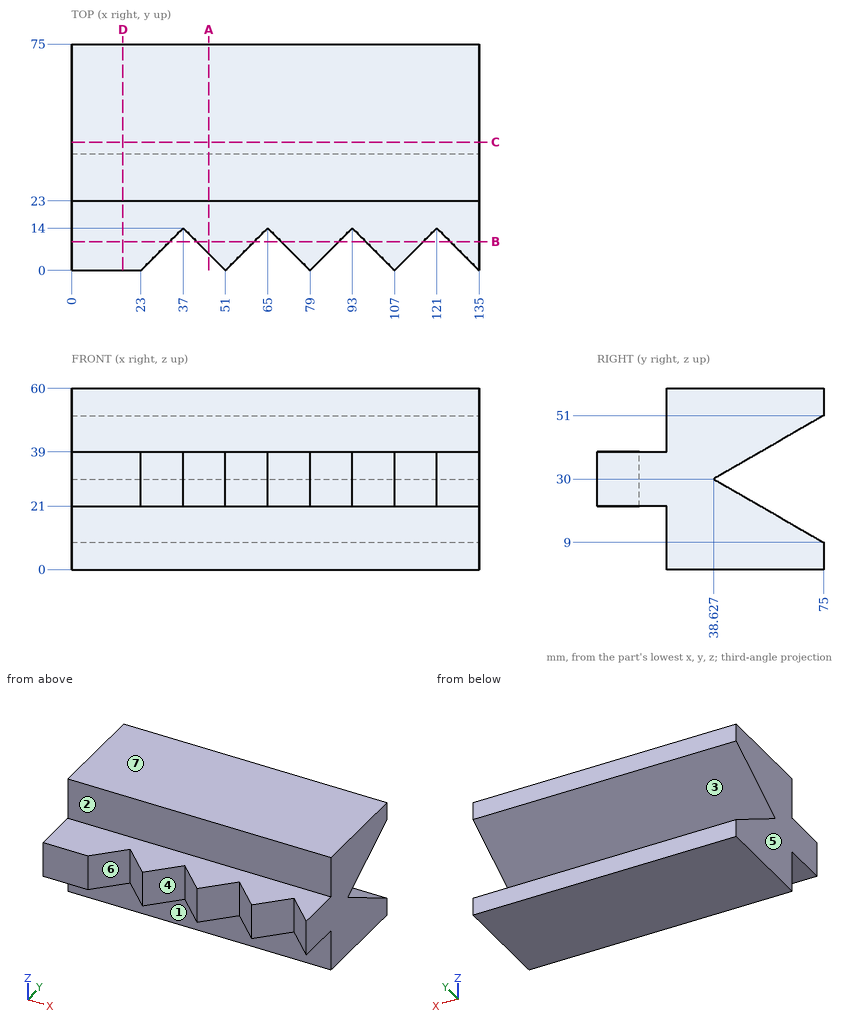
Source: three-view drawing plus pictorial views. Frame: mm from the lowest corner of the part. A direction names the side the tool comes from. Round coordinates to 2 decimals unless told otherwise and drop trailing zeros. Loops run counter-clockwise (first coordinate to the right, second up) from the corner with the lowest first, then second, coordinate; pieces in that order, holes last. Notation, with made-up numbers: M 45.25,75 L 98.25,75 A17 cw 98.25,100 Z; hole C 17,35.25 d9. An arc over 180 degrees is marked long. Put each result on its own line as item: value. Start each with the question number.
(1) Section query D-D (x = 17). Return loops of the section in (y, z).
(2) Material intervals for line 1 along Z through (x, y) = (22.5, 16); line 2 along Y through (x, z) = (11.5, 56); line 3 along Z through (x, y) = (55.5, 70), sorted ascending. Write a range as [from, to].
(3) Section query B-B (y = 9.5). Return loops of the section in (x, z), then the cut area to 3 significant figures.
(4) Section query C-C (y = 42.5). Return loops of the section in (x, z), then the cut area to 3 significant figures.
(5) Section query A-A (x = 45.5). Return loops of the section in (y, z).
(6) Draft query along X for the marked faces 4, 5, 6 and 7. Return one class per face: +X half, -X half, draft (parallel to the pull), parting line (faces both ways), or undercut.
(7) Contact query for flat-ended pins moving along their axis: pin 1 Ø1.5 at (x, y) = (93, 53.5) entering from -Z; pin 2 Ø10 at (x, z) = (62.5, 41) entering from -Y; pin 3 Ø17 at (x, z) = (70, 15.5) entering from -Y; pin 4 Ø10.5 at (x, z) = (81.5, 48) entering from -Y. Output: stop coordinate, or through.
(8) Set-up query: the marked faces 1, 2 and 3. Return all of +Z, -Z, +X, -X, +Y, -Y with unobstructed straight access to the full face (end or side cutting, diameter ignored); none if empty.
Findings below:
1. outline: M 0,21 L 23,21 L 23,0 L 75,0 L 75,9 L 38.63,30 L 75,51 L 75,60 L 23,60 L 23,39 L 0,39 Z
2. line 1: z = [21, 39]
2. line 2: y = [23, 75]
2. line 3: z = [0, 11.89], [48.11, 60]
3. outline: M 0,21 L 32.5,21 L 32.5,39 L 0,39 Z; M 41.5,21 L 60.5,21 L 60.5,39 L 41.5,39 Z; M 69.5,21 L 88.5,21 L 88.5,39 L 69.5,39 Z; M 97.5,21 L 116.5,21 L 116.5,39 L 97.5,39 Z; M 125.5,21 L 135,21 L 135,39 L 125.5,39 Z
3. area: 1,780 mm2
4. outline: M 0,0 L 135,0 L 135,27.76 L 0,27.76 Z; M 0,32.24 L 135,32.24 L 135,60 L 0,60 Z
4. area: 7,500 mm2
5. outline: M 5.5,21 L 23,21 L 23,0 L 75,0 L 75,9 L 38.63,30 L 75,51 L 75,60 L 23,60 L 23,39 L 5.5,39 Z
6. face 4: undercut
6. face 5: -X half
6. face 6: undercut
6. face 7: draft
7. pin 1: stops at z = 0
7. pin 2: stops at y = 6.92
7. pin 3: stops at y = 2.52
7. pin 4: stops at y = 23
8. face 1: -Z, +X, -X, -Y
8. face 2: +Z, +X, -X, -Y
8. face 3: +X, -X, +Y
